```python
from build123d import *
from OCP.BRepFilletAPI import BRepFilletAPI_MakeChamfer

# Parameters (mm, degrees)
EXTRUDE_2_DEPTH     = 2.5
SKETCH_4_W          = 3.5
SKETCH_4_H          = 2
SKETCH_4_H_2        = 3.5
CUT_EXTRUDE_1_DEPTH = 1
SKETCH_5_W          = 1.5
SKETCH_5_H          = 5
CUT_EXTRUDE_2_DEPTH = 1
SKETCH_6_W          = 0.7
SKETCH_6_H          = 0.7
EXTRUDE_3_DEPTH     = 3.5
CHAMFER_3_SIZE      = 0.2
CHAMFER_3_SIZE2     = 0.145308506


with BuildPart() as part:
    # Эскиз2 → Бобышка-Вытянуть2 (new, symmetric)
    with BuildSketch(Plane(origin=(0, 0, 0), x_dir=(0, -1, 0), z_dir=(1, 0, 0))):
        Polygon((0, -6.35), (0, 6.35), (-5.040100503, 7.95), (-13, -0.35), (-8, -6.35), align=None)
    extrude(amount=EXTRUDE_2_DEPTH, both=True)

    # Эскиз4 → Вырез-Вытянуть1 (cut)
    with BuildSketch(Plane(origin=(0, 6.5969489, -6.326632557), x_dir=(1, 0, 0), z_dir=(0, 0.7217391304347853, -0.6921651736393851))):
        with Locations((0, -7.250755953)):
            Rectangle(SKETCH_4_W, SKETCH_4_H)
        with Locations((0, -1.000755953)):
            Rectangle(SKETCH_4_W, SKETCH_4_H_2)
    extrude(amount=-CUT_EXTRUDE_1_DEPTH, mode=Mode.SUBTRACT)

    # Эскиз5 → Вырез-Вытянуть2 (cut)
    with BuildSketch(Plane(origin=(0, 7.844262295, 6.536885246), x_dir=(1, 0, 0), z_dir=(0, 0.7682212795973735, 0.6401843996644827))):
        with Locations((0.25, 3.243270072)):
            Rectangle(SKETCH_5_W, SKETCH_5_H)
    extrude(amount=-CUT_EXTRUDE_2_DEPTH, mode=Mode.SUBTRACT)

    # Эскиз6 → Бобышка-Вытянуть3 (add)
    with BuildSketch(Plane.XZ):
        with Locations((0.5, 1.35)):
            Rectangle(SKETCH_6_W, SKETCH_6_H)
        with Locations((0.5, -3.65)):
            Rectangle(SKETCH_6_W, SKETCH_6_H)
    extrude(amount=EXTRUDE_3_DEPTH)

    # Фаска3: one chamfer whose edges measure the first distance from different faces: ONE call of the kernel's chamfer builder (chamfer() names one face for all edges)
    chamfer_3_edges_1 = [part.edges().sort_by_distance(p)[0] for p in [
        (0.15, -3.5, 1.35),
    ]]
    chamfer_3_side_1 = [part.faces().sort_by_distance(p)[0] for p in [
        (0.15, -1.75, 1.35),
    ]]
    chamfer_3_edges_2 = [part.edges().sort_by_distance(p)[0] for p in [
        (0.5, -3.5, 1),
    ]]
    chamfer_3_side_2 = [part.faces().sort_by_distance(p)[0] for p in [
        (0.5, -1.75, 1),
    ]]
    chamfer_3_edges_3 = [part.edges().sort_by_distance(p)[0] for p in [
        (0.85, -3.5, 1.35),
    ]]
    chamfer_3_side_3 = [part.faces().sort_by_distance(p)[0] for p in [
        (0.85, -1.75, 1.35),
    ]]
    chamfer_3_edges_4 = [part.edges().sort_by_distance(p)[0] for p in [
        (0.5, -3.5, 1.7),
    ]]
    chamfer_3_side_4 = [part.faces().sort_by_distance(p)[0] for p in [
        (0.5, -1.75, 1.7),
    ]]
    chamfer_3_edges_5 = [part.edges().sort_by_distance(p)[0] for p in [
        (0.15, -3.5, -3.65),
    ]]
    chamfer_3_side_5 = [part.faces().sort_by_distance(p)[0] for p in [
        (0.15, -1.75, -3.65),
    ]]
    chamfer_3_edges_6 = [part.edges().sort_by_distance(p)[0] for p in [
        (0.5, -3.5, -4),
    ]]
    chamfer_3_side_6 = [part.faces().sort_by_distance(p)[0] for p in [
        (0.5, -1.75, -4),
    ]]
    chamfer_3_edges_7 = [part.edges().sort_by_distance(p)[0] for p in [
        (0.85, -3.5, -3.65),
    ]]
    chamfer_3_side_7 = [part.faces().sort_by_distance(p)[0] for p in [
        (0.85, -1.75, -3.65),
    ]]
    chamfer_3_edges_8 = [part.edges().sort_by_distance(p)[0] for p in [
        (0.5, -3.5, -3.3),
    ]]
    chamfer_3_side_8 = [part.faces().sort_by_distance(p)[0] for p in [
        (0.5, -1.75, -3.3),
    ]]
    chamfer_3 = BRepFilletAPI_MakeChamfer(part.part.solid().wrapped)
    for e in chamfer_3_edges_1:
        chamfer_3.Add(CHAMFER_3_SIZE, CHAMFER_3_SIZE2, e.wrapped, chamfer_3_side_1[0].wrapped)  # the first distance lies on this face
    for e in chamfer_3_edges_2:
        chamfer_3.Add(CHAMFER_3_SIZE, CHAMFER_3_SIZE2, e.wrapped, chamfer_3_side_2[0].wrapped)  # the first distance lies on this face
    for e in chamfer_3_edges_3:
        chamfer_3.Add(CHAMFER_3_SIZE, CHAMFER_3_SIZE2, e.wrapped, chamfer_3_side_3[0].wrapped)  # the first distance lies on this face
    for e in chamfer_3_edges_4:
        chamfer_3.Add(CHAMFER_3_SIZE, CHAMFER_3_SIZE2, e.wrapped, chamfer_3_side_4[0].wrapped)  # the first distance lies on this face
    for e in chamfer_3_edges_5:
        chamfer_3.Add(CHAMFER_3_SIZE, CHAMFER_3_SIZE2, e.wrapped, chamfer_3_side_5[0].wrapped)  # the first distance lies on this face
    for e in chamfer_3_edges_6:
        chamfer_3.Add(CHAMFER_3_SIZE, CHAMFER_3_SIZE2, e.wrapped, chamfer_3_side_6[0].wrapped)  # the first distance lies on this face
    for e in chamfer_3_edges_7:
        chamfer_3.Add(CHAMFER_3_SIZE, CHAMFER_3_SIZE2, e.wrapped, chamfer_3_side_7[0].wrapped)  # the first distance lies on this face
    for e in chamfer_3_edges_8:
        chamfer_3.Add(CHAMFER_3_SIZE, CHAMFER_3_SIZE2, e.wrapped, chamfer_3_side_8[0].wrapped)  # the first distance lies on this face
    add(Compound.cast(chamfer_3.Shape()), mode=Mode.REPLACE)


solid = part.part
```
Geometry: final body of the model. Coordinates: model frame, mm. A direction names the side the tool comes from. Give positions to 0.01 mm unless a question says otherwise; leave off trailing zeros. Order: outer loops, then holes, each group sorted by start corner. A loop starts at its lowest first (then second) coordinate and runs counter-clockwise, first axis right, second up. Notation, with made-up numbers: (-20, 74.25) -> (15, 74.25) arc R20 ccw to (15, 82.25) -> close; hole circle Ø7 at (-35.75, 83.5). An arc over 180 degrees is marked (long way). Write each question's results on one line, items separated by ' | '. Start each with the question number.
1) Section C-C (x = -1.5). Return loops of the section in (y, z), then the cut area to 3 significant figures.
2) First-contact query: pin 1 (0.8 mm diameter, centred on x = 0.5, y = -1, fed in from -Z); pin 2 (0.6 mm diameter, centred on y = -1, z = 1.5, fed in from -X); pin 3 (1 mm diameter, centred on x = -1, z = 4, fed in from -Y); pin 4 (8 mm diameter, centred on y = -1.5, z = 4.5, fed in from -X). Flat tips, straight axial feed; report the tip coordinate or a pass-through.
3) Section A-A (y = -0.25). Return loops of the section in (x, z), then the cut area to 3 significant figures.
4) Set-up query: faces 1 (the flat face through (0.24, 9.175, 3.378)), 2 (the flat face through (0.035, 2.485, -7.139)). Return all of +Z, -Z, +X, -X, +Y, -Y with unobstructed straight access to the full face (end or side cutting, diameter ignored); none if empty.
5) Line query: line 1 (X direction, y = 8.25, z = 4.75); line 2 (X direction, y = 6, z = -6.75); line 3 (Z direction, x = 0.25, y = 5.75). Output: solid intervals per line, ascending. Write a range as from..to.
6) Section B-B (z = 0). Return loops of the section in (x, y).
7) Draft query along X for faces 3 (the flat face through (-2.5, 5, -1)), 4 (the flat face through (-1.75, 7, -5)), 5 (the flat face through (0, 4, 6.35)), 6 (the flat face through (-0.024, 10.884, -0.411)). Return one class per face: pulls with the +X half, pulls with the -X half, needs draft (parallel to the pull), parting line crosses it, or undercut.
8) Section D-D (y = 11.25). Return loops of the section in (x, z), then the cut area to 3 significant figures.
Calculated:
1) outline: (0, -6.35) -> (5.04, -7.95) -> (6.08, -6.87) -> (5.36, -6.18) -> (7.78, -3.65) -> (8.5, -4.34) -> (10.92, -1.82) -> (10.2, -1.12) -> (11.59, 0.32) -> (12.31, -0.37) -> (13, 0.35) -> (8, 6.35) -> (0, 6.35) -> close | area: 128 mm2
2) pin 1: z = -4 | pin 2: x = 0.15 | pin 3: y = 0 | pin 4: x = -2.5
3) outline: (0.15, -4) -> (0.85, -4) -> (0.85, -3.3) -> (0.15, -3.3) -> close; (0.15, 1) -> (0.85, 1) -> (0.85, 1.7) -> (0.15, 1.7) -> close | area: 0.980 mm2
4) face 1: none | face 2: -Z, +X, -X, -Y
5) line 1: -2.5..-0.5, 1..2.5 | line 2: -2.5..-1.75, 1.75..2.5 | line 3: -7.21..-6.55, -5.77..6.35
6) outline: (-2.5, 0) -> (2.5, 0) -> (2.5, 12.66) -> (-2.5, 12.66) -> close; hole (-1.75, 11.28) -> (1.75, 11.28) -> (1.75, 11.92) -> (-1.75, 11.92) -> close
7) face 3: pulls with the -X half | face 4: undercut | face 5: needs draft | face 6: undercut
8) outline: (-2.5, -1.47) -> (-1.75, -1.47) -> (-1.75, -0.03) -> (1.75, -0.03) -> (1.75, -1.47) -> (2.5, -1.47) -> (2.5, 2.45) -> (1, 2.45) -> (1, 1.9) -> (-0.5, 1.9) -> (-0.5, 2.45) -> (-2.5, 2.45) -> close | area: 13.7 mm2
